The figure shows three views and two pictorial views of one solid part (mm, origin at its lowest corner). Answer the questions. Round coordinates to 2 decimals unless told otherwise and drop trailing zeros. Order: outer loops, then holes, each group sorted by start corner. A loop starts at its lowest first (then second) coordinate and runs counter-clockwise, first axis right, second up. Notation, with made-up numbers: M -19,70.25 L 33,70.25 A18 cw 33,91.25 Z; hole C -19,41.25 d3. An arc over 180 degrees is marked long. Return JSON: item names as keys, results as strings.
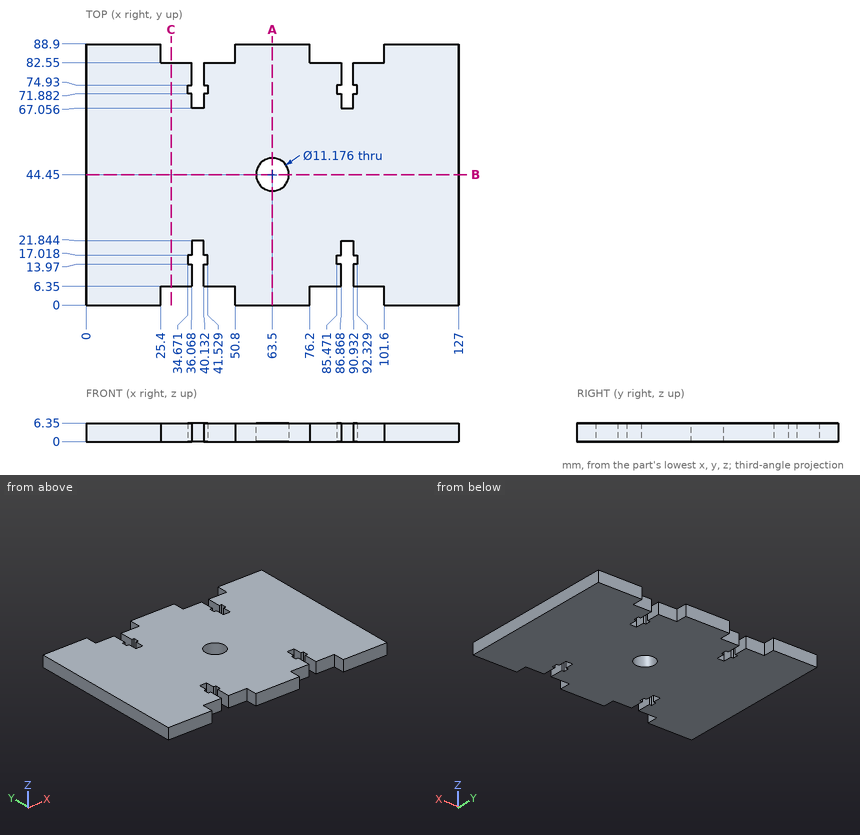
Item 1: Find section A-A (x = 63.5). Determine the outline of the cut face in (y, z), plus the area to 3 significant figures.
Output:
{"outline": "M 0,0 L 38.86,0 L 38.86,6.35 L 0,6.35 Z; M 50.04,0 L 88.9,0 L 88.9,6.35 L 50.04,6.35 Z", "area": "494 mm^2"}
Item 2: Consider line 1 along X through (y, z) = (5.5, 0.5); line 2 along X through (y, z) = (12.5, 2); line 3 along Y through (x, z) = (63.5, 5.25). Determine where each line is inside the solid, lowest interval first. Write a range as [from, to].
Output:
{"line 1": "x = [0, 25.4], [50.8, 76.2], [101.6, 127]", "line 2": "x = [0, 36.07], [40.13, 86.87], [90.93, 127]", "line 3": "y = [0, 38.86], [50.04, 88.9]"}
Item 3: Find section C-C (x = 29). Determine the outline of the cut face in (y, z), plus the area to 3 significant figures.
Output:
{"outline": "M 6.35,0 L 82.55,0 L 82.55,6.35 L 6.35,6.35 Z", "area": "484 mm^2"}
Item 4: Each of these flat-tipped pins is pushed along its axis until it touches: pin 1 (1.5 mm diameter, centred on x = 35.5, z = 3, fed in from +Y); pin 2 (1.5 mm diameter, centred on x = 86.5, z = 4.5, fed in from -Y); pin 3 (2.5 mm diameter, centred on y = 19, z = 2.5, fed in from -X). Where does it stop, or does it pass through?
Output:
{"pin 1": "stops at y = 82.55", "pin 2": "stops at y = 6.35", "pin 3": "stops at x = 0"}
Item 5: Find section B-B (y = 44.45). Determine the outline of the cut face in (x, z), plus the area to 3 significant figures.
Output:
{"outline": "M 0,0 L 57.91,0 L 57.91,6.35 L 0,6.35 Z; M 69.09,0 L 127,0 L 127,6.35 L 69.09,6.35 Z", "area": "735 mm^2"}
